from build123d import *

# Parameters (mm, degrees)
F0_W                 = 175
F0_H                 = 85
F0_R                 = 2.25
F0_R_2               = 1.15
F1_DEPTH             = 2
F2_D                 = 4.3
F4_D                 = 2.3
F4_CSINK_D           = 4.5
F4_CSINK_ANGLE       = 90
F4_ON_F3_D           = 2.3
F4_ON_F3_CSINK_D     = 4.5
F4_ON_F3_CSINK_ANGLE = 90


# Not quite as in the source:
# - ends of sketch curves that miss each other by under 0.0002 mm in the source are joined


with BuildPart() as f1:
    # F0 (on Top) → F1 (new body)
    with BuildSketch(Plane.XY):
        Rectangle(F0_W, F0_H)
        with BuildLine():
            ThreePointArc((-80.499999, -37.5), (-82.499999, -39.5), (-84.499999, -37.5))
            ThreePointArc((-84.499999, -37.5), (-82.4999995, -35.499999), (-80.499999, -37.5))
        make_face(mode=Mode.SUBTRACT)
        with Locations((-72.5, -40)):
            Circle(F0_R, mode=Mode.SUBTRACT)
        with Locations((-85, -32)):
            Circle(F0_R, mode=Mode.SUBTRACT)
        with Locations((-32.5, -40)):
            Circle(F0_R, mode=Mode.SUBTRACT)
        with Locations((7.5, -40)):
            Circle(F0_R, mode=Mode.SUBTRACT)
        with BuildLine():
            ThreePointArc((19.500001, -37.5), (17.500001, -39.5), (15.500001, -37.5))
            ThreePointArc((15.500001, -37.5), (17.5000005, -35.499999), (19.500001, -37.5))
        make_face(mode=Mode.SUBTRACT)
        with Locations((27.5, -40)):
            Circle(F0_R, mode=Mode.SUBTRACT)
        with Locations((67.5, -40)):
            Circle(F0_R, mode=Mode.SUBTRACT)
        with BuildLine():
            ThreePointArc((84.500001, -37.5), (82.500001, -39.5), (80.500001, -37.5))
            ThreePointArc((80.500001, -37.5), (82.5000005, -35.499999), (84.500001, -37.5))
        make_face(mode=Mode.SUBTRACT)
        with Locations((85, -27.5)):
            Circle(F0_R, mode=Mode.SUBTRACT)
        with Locations((-85, 0)):
            Circle(F0_R, mode=Mode.SUBTRACT)
        with Locations((-85, 27.5)):
            Circle(F0_R, mode=Mode.SUBTRACT)
        with BuildLine():
            ThreePointArc((-80.499999, 37.5), (-82.499999, 35.5), (-84.499999, 37.5))
            ThreePointArc((-84.499999, 37.5), (-82.4999995, 39.500001), (-80.499999, 37.5))
        make_face(mode=Mode.SUBTRACT)
        with Locations((-72.5, 40)):
            Circle(F0_R, mode=Mode.SUBTRACT)
        with Locations((-32.5, 40)):
            Circle(F0_R, mode=Mode.SUBTRACT)
        with Locations((85, 0)):
            Circle(F0_R, mode=Mode.SUBTRACT)
        with Locations((7.5, 40)):
            Circle(F0_R, mode=Mode.SUBTRACT)
        with BuildLine():
            ThreePointArc((19.500001, 37.5), (17.500001, 35.5), (15.500001, 37.5))
            ThreePointArc((15.500001, 37.5), (17.5000005, 39.500001), (19.500001, 37.5))
        make_face(mode=Mode.SUBTRACT)
        with Locations((27.5, 40)):
            Circle(F0_R, mode=Mode.SUBTRACT)
        with Locations((85, 24.3)):
            Circle(F0_R, mode=Mode.SUBTRACT)
        with Locations((67.5, 40)):
            Circle(F0_R, mode=Mode.SUBTRACT)
        with BuildLine():
            ThreePointArc((84.500001, 37.5), (82.500001, 35.5), (80.500001, 37.5))
            ThreePointArc((80.500001, 37.5), (82.5000005, 39.500001), (84.500001, 37.5))
        make_face(mode=Mode.SUBTRACT)
        with Locations((-85, 27.5)):
            Circle(F0_R)
        with Locations((-85, 27.5)):
            Circle(F0_R_2, mode=Mode.SUBTRACT)
        with Locations((7.5, 40)):
            Circle(F0_R)
        with Locations((7.5, 40)):
            Circle(F0_R_2, mode=Mode.SUBTRACT)
        with Locations((-32.5, -40)):
            Circle(F0_R)
        with Locations((-32.5, -40)):
            Circle(F0_R_2, mode=Mode.SUBTRACT)
        with Locations((7.5, -40)):
            Circle(F0_R)
        with Locations((7.5, -40)):
            Circle(F0_R_2, mode=Mode.SUBTRACT)
        with Locations((-85, 0)):
            Circle(F0_R)
        with Locations((-85, 0)):
            Circle(F0_R_2, mode=Mode.SUBTRACT)
        with Locations((-32.5, 40)):
            Circle(F0_R)
        with Locations((-32.5, 40)):
            Circle(F0_R_2, mode=Mode.SUBTRACT)
        with Locations((85, 0)):
            Circle(F0_R)
        with Locations((85, 0)):
            Circle(F0_R_2, mode=Mode.SUBTRACT)
        with Locations((-72.5, 40)):
            Circle(F0_R)
        with Locations((-72.5, 40)):
            Circle(F0_R_2, mode=Mode.SUBTRACT)
        with Locations((-85, -32)):
            Circle(F0_R)
        with Locations((-85, -32)):
            Circle(F0_R_2, mode=Mode.SUBTRACT)
        with Locations((-72.5, -40)):
            Circle(F0_R)
        with Locations((-72.5, -40)):
            Circle(F0_R_2, mode=Mode.SUBTRACT)
        with Locations((27.5, 40)):
            Circle(F0_R)
        with Locations((27.5, 40)):
            Circle(F0_R_2, mode=Mode.SUBTRACT)
        with Locations((27.5, -40)):
            Circle(F0_R)
        with Locations((27.5, -40)):
            Circle(F0_R_2, mode=Mode.SUBTRACT)
        with Locations((67.5, 40)):
            Circle(F0_R)
        with Locations((67.5, 40)):
            Circle(F0_R_2, mode=Mode.SUBTRACT)
        with Locations((85, 24.3)):
            Circle(F0_R)
        with Locations((85, 24.3)):
            Circle(F0_R_2, mode=Mode.SUBTRACT)
        with Locations((67.5, -40)):
            Circle(F0_R)
        with Locations((67.5, -40)):
            Circle(F0_R_2, mode=Mode.SUBTRACT)
        with Locations((85, -27.5)):
            Circle(F0_R)
        with Locations((85, -27.5)):
            Circle(F0_R_2, mode=Mode.SUBTRACT)
        with BuildLine():
            ThreePointArc((-80.499999, -37.499999), (-82.4999995, -35.499999), (-84.499999, -37.5))
            ThreePointArc((-84.499999, -37.5), (-82.499999, -39.5), (-80.499999, -37.499999))
        make_face()
        with BuildLine():
            ThreePointArc((19.500001, -37.499999), (17.5000005, -35.499999), (15.500001, -37.5))
            ThreePointArc((15.500001, -37.5), (17.500001, -39.5), (19.500001, -37.499999))
        make_face()
        with BuildLine():
            ThreePointArc((84.500001, 37.500001), (82.5000005, 39.500001), (80.500001, 37.5))
            ThreePointArc((80.500001, 37.5), (82.500001, 35.5), (84.500001, 37.500001))
        make_face()
        with BuildLine():
            ThreePointArc((19.500001, 37.500001), (17.5000005, 39.500001), (15.500001, 37.5))
            ThreePointArc((15.500001, 37.5), (17.500001, 35.5), (19.500001, 37.500001))
        make_face()
        with BuildLine():
            ThreePointArc((-80.499999, 37.500001), (-82.4999995, 39.500001), (-84.499999, 37.5))
            ThreePointArc((-84.499999, 37.5), (-82.499999, 35.5), (-80.499999, 37.500001))
        make_face()
        with BuildLine():
            ThreePointArc((84.500001, -37.499999), (82.5000005, -35.499999), (80.500001, -37.5))
            ThreePointArc((80.500001, -37.5), (82.500001, -39.5), (84.500001, -37.499999))
        make_face()
        with Locations((-85, 27.5)):
            Circle(F0_R_2)
        with Locations((85, 24.3)):
            Circle(F0_R_2)
        with Locations((-85, -32)):
            Circle(F0_R_2)
        with Locations((-72.5, -40)):
            Circle(F0_R_2)
        with Locations((-32.5, -40)):
            Circle(F0_R_2)
        with Locations((7.5, -40)):
            Circle(F0_R_2)
        with Locations((-72.5, 40)):
            Circle(F0_R_2)
        with Locations((7.5, 40)):
            Circle(F0_R_2)
        with Locations((-32.5, 40)):
            Circle(F0_R_2)
        with Locations((85, 0)):
            Circle(F0_R_2)
        with Locations((27.5, -40)):
            Circle(F0_R_2)
        with Locations((-85, 0)):
            Circle(F0_R_2)
        with Locations((67.5, 40)):
            Circle(F0_R_2)
        with Locations((27.5, 40)):
            Circle(F0_R_2)
        with Locations((67.5, -40)):
            Circle(F0_R_2)
        with Locations((85, -27.5)):
            Circle(F0_R_2)
    extrude(amount=-F1_DEPTH)

    # F2 (through all)
    with Locations(Plane.XY):
        with Locations((-82.499999, 37.5), (17.500001, 37.5), (82.500001, 37.5), (82.500001, -37.5), (-82.499999, -37.5), (17.500001, -37.5)):
            Hole(F2_D / 2)

    # F4 (through all)
    with Locations(Plane.XY):
        with Locations((-85, -32), (-72.5, -40), (-85, 27.5), (-72.5, 40), (-32.5, -40), (7.5, -40), (27.5, -40), (67.5, -40), (-32.5, 40), (7.5, 40), (27.5, 40), (67.5, 40), (85, -27.5)):
            CounterSinkHole(F4_D / 2, F4_CSINK_D / 2, counter_sink_angle=F4_CSINK_ANGLE)

    # F4 on F3 (through all)
    with Locations(Plane.XY):
        with Locations((85, 32), (85, 2.25), (-85, 1.2), (-27.35, 1), (29.35, 1)):
            CounterSinkHole(F4_ON_F3_D / 2, F4_ON_F3_CSINK_D / 2, counter_sink_angle=F4_ON_F3_CSINK_ANGLE)


solid = f1.part
Model file for the job. Use its own axes, mm. Give positions to 0.01 mm unless a question says otherwise; leave off trailing zeros. One line per item, written item: value.
Item 1: Wall check: line 1 (Y direction, x = 67.5, z = -1.5); line 2 (X direction, y = -40, z = -1.6); line 3 (Y direction, x = 82.5, z = -0.45). Give the ranges that are in metal, low to high.
Response values:
line 1: -42.5 to -41.15, -38.85 to 38.85, 41.15 to 42.5
line 2: -87.5 to -73.65, -71.35 to -33.65, -31.35 to 6.35, 8.65 to 26.35, 28.65 to 66.35, 68.65 to 87.5
line 3: -42.5 to -39.65, -35.35 to 35.35, 39.65 to 42.5
Item 2: Two-plate mould, pull along X, no slides. Class faces 1 (the cylindrical face through (-82.22, 39.63, -1.01)), 2 (the flat face through (-1, 1, 0)): released by +X, released by -X, zero draft, split by the parting line, or undercut.
Response values:
face 1: undercut
face 2: zero draft
Item 3: Pin check, flat tips, straight feed: pin 1 Ø3 at (x, y) = (-85, 1.2) entering from -Z; pin 2 Ø3.5 at (x, y) = (27.5, -40) entering from +Z; pin 3 Ø3 at (x, y) = (67.5, -40) entering from +Z; pin 4 Ø2.5 at (x, y) = (-72.5, -40) entering from +Z. Stop position of each tip, or through.
Response values:
pin 1: z = -2
pin 2: z = -0.5
pin 3: z = -0.75
pin 4: z = -1
